Check sheet for the modelled part. Datum: model origin and axes. Units: mm. Round coordinates to 2 decimals unless told otherwise and drop trailing zeros. Loops run counter-clockwise (first coordinate to the right, second up) from the corner with the lowest first, then second, coordinate; pieces in that order, holes last. Notation, with made-up numbers: (29, 45.25) -> (61, 45.25) arc R19 cw to (61, 51.25) -> close; hole circle Ø5 at (77, 73.25). An arc over 180 degrees is marked (long way). Return JSON: item names as keys, results as strings.
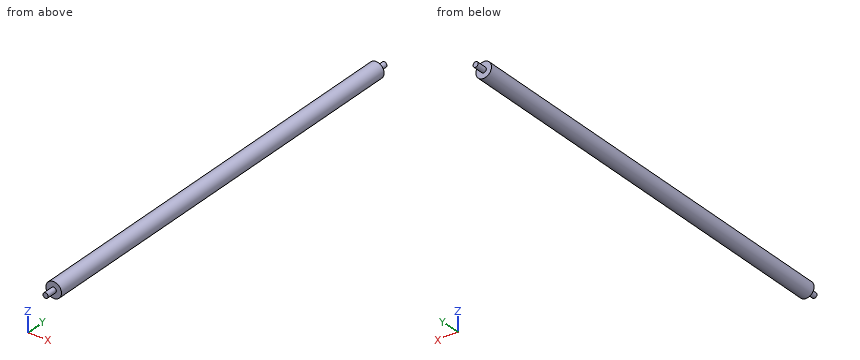
from build123d import *

# Parameters (mm, degrees)
F0_R     = 15
F0_R_2   = 5
F1_DEPTH = 800
F2_DEPTH = 20
F4_R     = 5
F5_DEPTH = 20


with BuildPart() as f1:
    # F0 (on Front) → F1 (new body)
    with BuildSketch(Plane.XZ):
        Circle(F0_R)
        Circle(F0_R_2, mode=Mode.SUBTRACT)
        Circle(F0_R_2)
    extrude(amount=F1_DEPTH)

    # F0 (on Front) → F2 (join)
    with BuildSketch(Plane.XZ):
        Circle(F0_R_2)
    extrude(amount=-F2_DEPTH)

    # F4 (on offset) → F5 (join)
    with BuildSketch(Plane.XZ.offset(800)):
        Circle(F4_R)
    extrude(amount=F5_DEPTH)


solid = f1.part
Q1. Go/stop test with flat-tipped pins: pin 1 (4 mm diameter, centred on y = -701, z = 5.5, fed in from -X); pin 2 (1.5 mm diameter, centred on x = 5, z = 11.5, fed in from -Y); pin 3 (12 mm diameter, centred on x = -9.5, y = -271, fed in from +Z); pin 4 (4 mm diameter, centred on y = -500, z = -0.5, fed in from +X). Record where each tip stops, or that it passes through.
Results list:
{"pin 1": "x = -14.59", "pin 2": "y = -800", "pin 3": "z = 14.59", "pin 4": "x = 15"}
Q2. Section check C-C (y = -133). Record the boundary of the cut face in (x, z).
Results list:
{"outline": "circle Ø30 at (0, 0)"}
Q3. Section check A-A (z = 0). Record the boundary of the cut face in (x, y), then the cut area to 3 significant figures.
Results list:
{"outline": "(-15, -800) -> (-5, -800) -> (-5, -820) -> (5, -820) -> (5, -800) -> (15, -800) -> (15, 0) -> (5, 0) -> (5, 20) -> (-5, 20) -> (-5, 0) -> (-15, 0) -> close", "area": "24,400 mm^2"}
Q4. Section check B-B (x = 0). Record the boundary of the cut face in (y, z), then the cut area to 3 significant figures.
Results list:
{"outline": "(-820, -5) -> (-800, -5) -> (-800, -15) -> (0, -15) -> (0, -5) -> (20, -5) -> (20, 5) -> (0, 5) -> (0, 15) -> (-800, 15) -> (-800, 5) -> (-820, 5) -> close", "area": "24,400 mm^2"}
Q5. Material ranges on line 1 (Y direction, x = 2, z = 9); line 2 (X direction, y = -430, z = 1); line 3 (Z direction, x = -0.5, y = -328), recorded low to high.
Results list:
{"line 1": "-800 to 0", "line 2": "-14.97 to 14.97", "line 3": "-14.99 to 14.99"}
